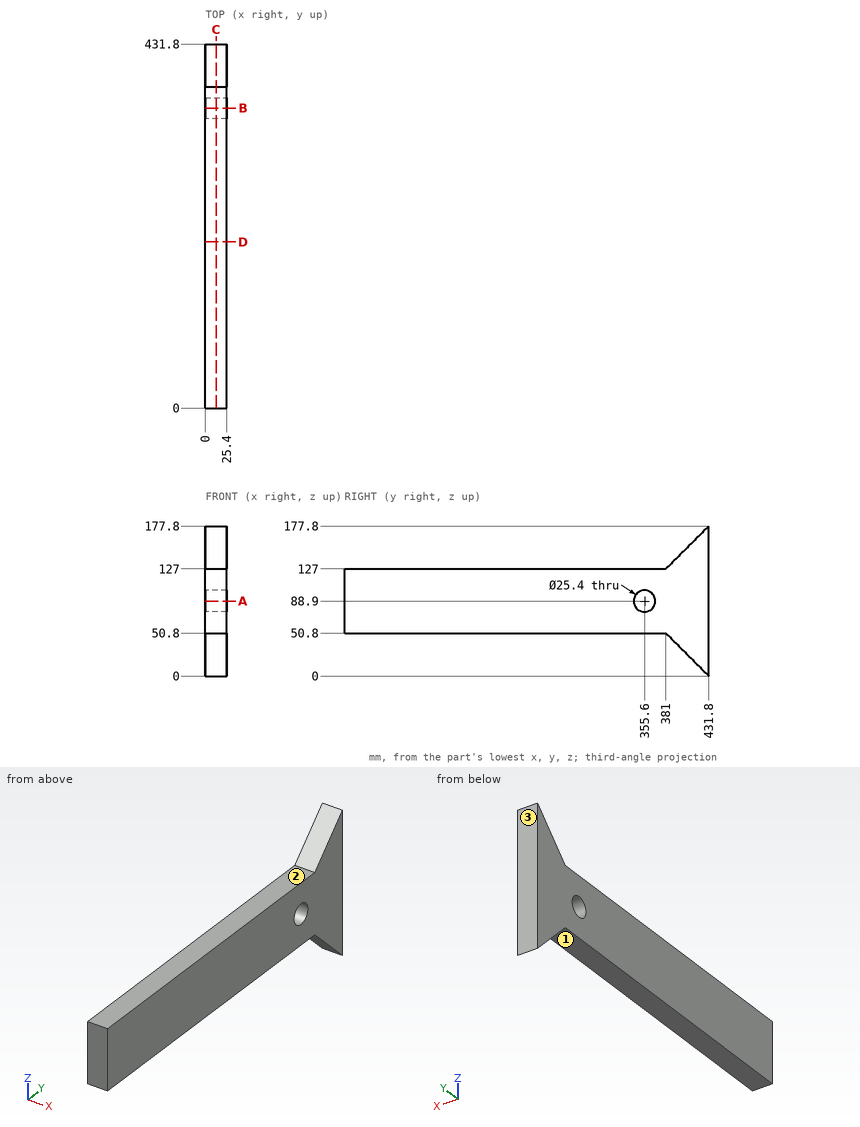
The drawing under review shows one solid part. Ordinate dimensions are in mm from its lowest x, y, z. A direction names the side the tool comes from. Coordinates: 2 decimals unless noted, no trailing zeros. Write each loop counter-clockwise with the first axis right and the second up, starting at its lowest first coordinate (ties: lowest second). Pieces come first, ordered by that corner, then holes. Notation, with made-up numbers: (55.25, 58) - (90.25, 58) arc R5 ccw to (90.25, 63) - close; hole circle Ø8 at (23, 88). An arc over 180 degrees is marked (long way). Answer in a Markdown table with one row per item. Add a question column.
Q1. We need section B-B, the plane y = 355.6. State the section outline as (x, z) points.
Q2. For probe 1 along Z at (x, y) = (8.75, 355.6); probe 2 along Z at (x, y) = (13.25, 166); probe 3 along Y at (x, z) = (18.75, 17), list the stretches that pass through material, from the lowest coordinate up.
Q3. For P1, Ø10, axis at x = 3.5, y = 134.5, coming from the -Z side; P2, Ø2, axis at x = 3, y = 358, coming from the +Z side; P3, Ø8, axis at y = 356, z = 132, coming from the +X side, all flat-tipped, find the tip position at first contact; note any pin that passes through.
Q4. We need section D-D, the plane y = 197. State the section outline as (x, z) points, and give its area (3 significant figures).
Q5. Tool access review of the marked faces 1, 2 and 3: name each direction out of +Z, -Z, +X, -X, +Y, -Y from which nothing blocks a thin tool from reaching the whole face with its end or side.
Q6. We need section C-C, the plane x = 13. State the section outline as (y, z) points, and give its area (3 significant figures).
Q7. We need section A-A, the plane z = 88.9. State the section outline as (x, y) points.
Answer list:
| question | item | result |
|---|---|---|
| 1 | outline | (0, 50.8) - (25.4, 50.8) - (25.4, 76.2) - (0, 76.2) - close; (0, 101.6) - (25.4, 101.6) - (25.4, 127) - (0, 127) - close |
| 2 | probe 1 | z = 50.8 to 76.2, 101.6 to 127 |
| 2 | probe 2 | z = 50.8 to 127 |
| 2 | probe 3 | y = 414.8 to 431.8 |
| 3 | P1 | stops at z = 50.8 |
| 3 | P2 | stops at z = 127 |
| 3 | P3 | passes through |
| 4 | outline | (0, 50.8) - (25.4, 50.8) - (25.4, 127) - (0, 127) - close |
| 4 | area | 1,940 mm2 |
| 5 | face 1 | -Z, +X, -X, -Y |
| 5 | face 2 | +Z, +X, -X, -Y |
| 5 | face 3 | +Z, -Z, +X, -X, +Y |
| 6 | outline | (0, 50.8) - (381, 50.8) - (431.8, 0) - (431.8, 177.8) - (381, 127) - (0, 127) - close; hole circle Ø25.4 at (355.6, 88.9) |
| 6 | area | 35,000 mm2 |
| 7 | outline | (0, 0) - (25.4, 0) - (25.4, 342.9) - (0, 342.9) - close; (0, 368.3) - (25.4, 368.3) - (25.4, 431.8) - (0, 431.8) - close |
